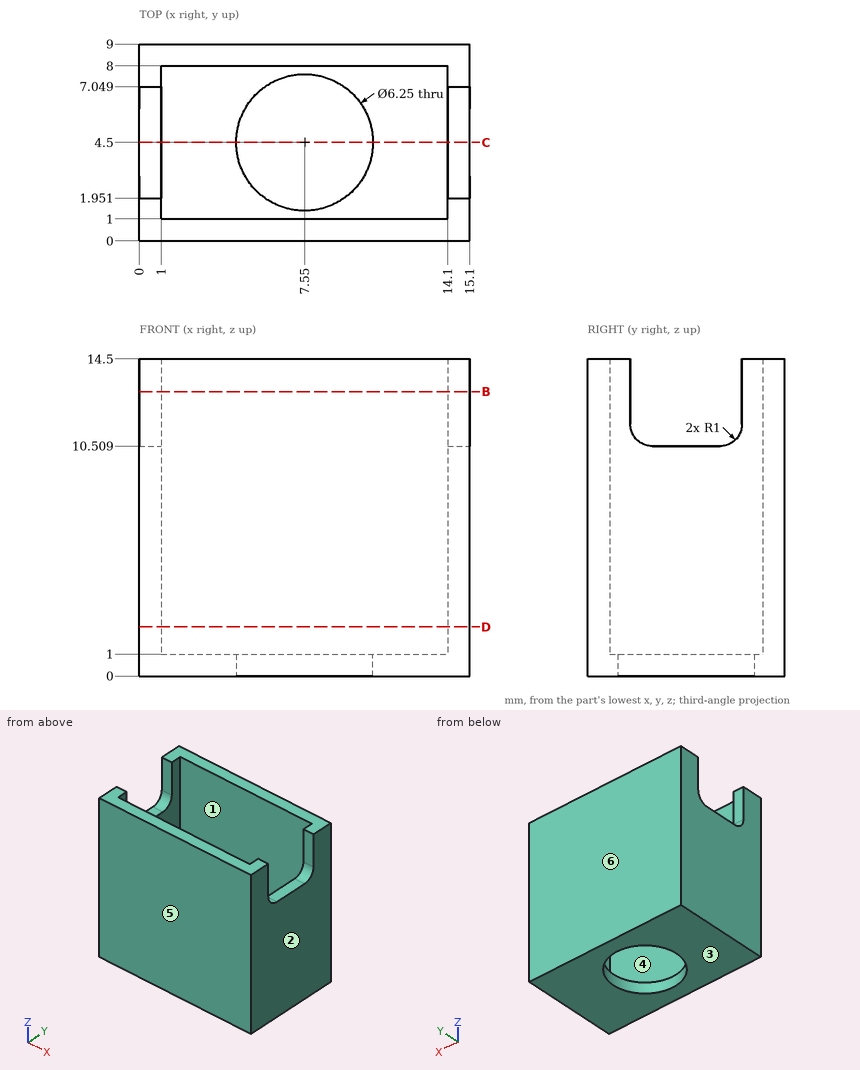
The figure shows three views and two pictorial views of one solid part (mm, origin at its lowest corner). Answer the questions. A direction names the side the tool comes from. Coordinates: 2 decimals unless noted, no trailing zeros. Loops run counter-clockwise (first coordinate to the right, second up) from the corner with the lowest first, then second, coordinate; pieces in that order, holes last. Notation, with made-up numbers: M 39,62 L 45,62 A19 ccw 45,69 Z; hole C 39.25,-14 d4. An arc over 180 degrees is marked long. Use CSV: the item, a comma, the result in double quotes. Start each with the question number.
(1) Find section D-D, the plane z = 2.25. Give the vertices of the cut face in (x, y).
(2) Find section C-C, the plane y = 4.5. Give the vertices of the cut face in (x, z) (1 decimal).
(3) For a pull along Y with two mould halves and no side action, classify the marked faces 3, 4, 5 and 6 as +Y half, -Y half, draft (parallel to the pull), parting line (faces both ways), or undercut.
(4) Find section B-B, the plane z = 13. Give the vertices of the cut face in (x, y).
(5) For the marked faces 1 and 2, determine the directions among +Z, -Z, +X, -X, +Y, -Y from which every point of the face is accessible in a straight line to the end or side of a thin tool.
(6) Consider line 1 (Y direction, x = 7.55, z = 0.3) (1 decimal); line 2 (Y direction, x = 8.25, z = 8.25); line 3 (X direction, y = 3, z = 5.5). Determine where each line is inside the solid, lowest interval first.
(7) Given pin 1 Ø3.5 at (x, y) = (7, 4) entering from +Z; pin 2 Ø5 at (y, z) = (8, 9) entering from -X; pin 3 Ø1.1 at (x, y) = (14.5, 4) entering from +Z, each flat-ended and moving along its own axis, determine where each tip first touches the part or whether it passes through.
Recorded:
1,outline,"M 0,0 L 15.1,0 L 15.1,9 L 0,9 Z; hole M 1,1 L 14.1,1 L 14.1,8 L 1,8 Z"
2,outline,"M 0,0 L 4.4,0 L 4.4,1 L 1,1 L 1,10.5 L 0,10.5 Z; M 10.7,0 L 15.1,0 L 15.1,10.5 L 14.1,10.5 L 14.1,1 L 10.7,1 Z"
3,face 3,"draft"
3,face 4,"undercut"
3,face 5,"-Y half"
3,face 6,"+Y half"
4,outline,"M 0,0 L 15.1,0 L 15.1,1.95 L 14.1,1.95 L 14.1,1 L 1,1 L 1,1.95 L 0,1.95 Z; M 0,7.05 L 1,7.05 L 1,8 L 14.1,8 L 14.1,7.05 L 15.1,7.05 L 15.1,9 L 0,9 Z"
5,face 1,"+Z"
5,face 2,"+Z, -Z, +X, +Y, -Y"
6,line 1,"y = 0 to 1.4, 7.6 to 9"
6,line 2,"y = 0 to 1, 8 to 9"
6,line 3,"x = 0 to 1, 14.1 to 15.1"
7,pin 1,"passes through"
7,pin 2,"stops at x = 0"
7,pin 3,"stops at z = 10.51"
